The figure shows three views and two pictorial views of one solid part (mm, origin at its lowest corner). Answer the questions. A direction names the side the tool comes from. Give positions to 0.01 mm unless a question says otherwise; leave off trailing zeros. Order: outer loops, then holes, each group sorted by start corner. A loop starts at its lowest first (then second) coordinate and runs counter-clockwise, first axis right, second up. Notation, with made-up numbers: (25, 6) - (39, 6) arc R22 cw to (39, 35) - close; hole circle Ø1 at (-39.5, 58). An arc over 180 degrees is marked (long way). Write item = value, one per line.
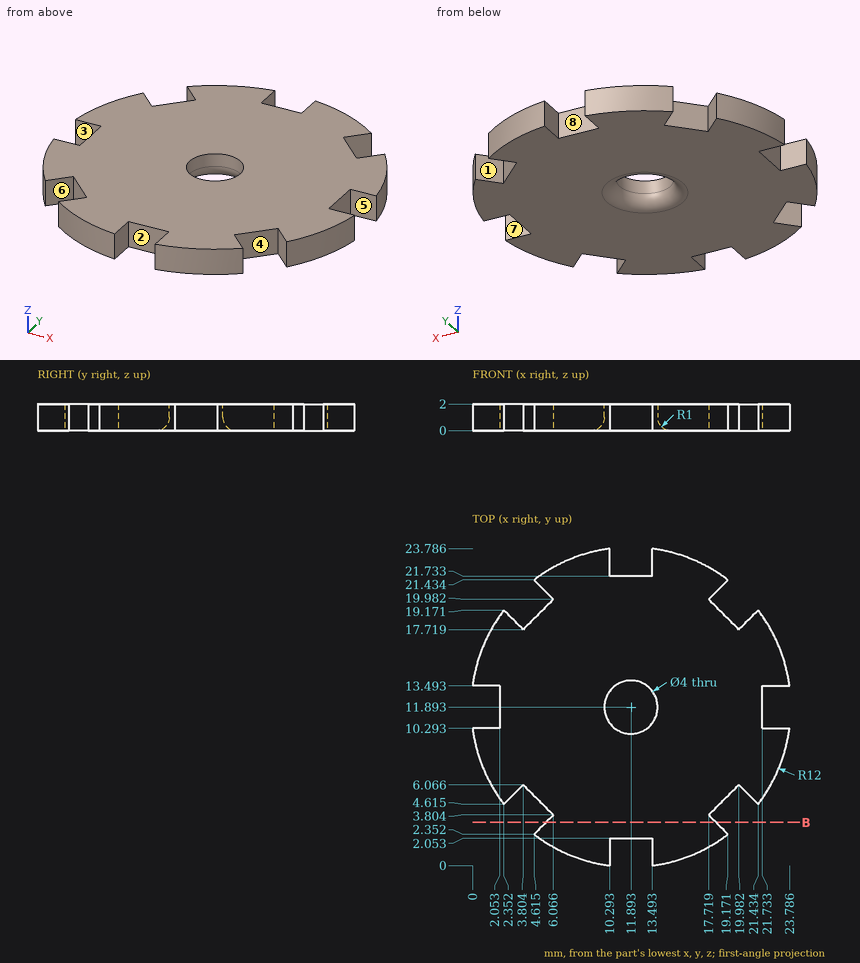
1. Straight lines are drawn through the part: L1, parallel to Y at x = 19, z = 1 (1 decimal); L2, parallel to Y at x = 18, z = 0.55 (1 decimal); L3, parallel to Y at x = 10.5, z = 0.7 (1 decimal). For each, find the intervals that lie inside material, in ascending order. Write a range as [from, to].
Recorded:
L1 = [2.2, 2.5], [5.1, 18.7], [21.3, 21.6]
L2 = [1.6, 3.5], [4.1, 19.7], [20.3, 22.2]
L3 = [2.1, 10.4], [13.4, 21.7]
2. For the marked faces 1, 2, 3, 4 and 5, determine the directions among +Z, -Z, +X, -X, +Y, -Y from which every point of the face is accessible in a straight line to the end or side of a thin tool.
Recorded:
face_1 = +Z, -Z, +Y
face_2 = +Z, -Z, -Y
face_3 = +Z, -Z, -X
face_4 = +Z, -Z
face_5 = +Z, -Z, +X
3. Determine the mould class of the marked faces 6, 7 and 8 for opening direction Y: +Y half, -Y half, draft (parallel to the pull), parting line (faces both ways), or undercut.
Recorded:
face_6 = -Y half
face_7 = undercut
face_8 = +Y half
4. Flat-ended cylindrical pins translate along their axes: pin 1 (0.6 mm diameter, centred on y = 23, z = 1, fed in from +X); pin 2 (1 mm diameter, centred on x = 22.5, z = 1.5, fed in from +Y); pin 3 (0.6 mm diameter, centred on x = 11.5, z = 0.5, fed in from -Y). Find the tip coordinate at first contact, or state that the pin passes through.
Recorded:
pin_1 = 17.11
pin_2 = 18.36
pin_3 = 2.05
5. Section B-B (y = 3.25) is taken. Determine the outline of the cut face in (x, z).
Recorded:
outline = (5.51, 0) - (18.27, 0) - (18.27, 2) - (5.51, 2) - close
